Read the model definition and answer for the solid it produces. Units are mm, in the model's axes. Face numbers are marked on the shaded views. Give positions to 0.01 mm unless a question says otherwise; leave off trailing zeros. Order: outer loops, then holes, each group sorted by start corner. A loop starts at its lowest first (then second) coordinate and runs counter-clockwise, first axis right, second up. Notation, with made-up numbers: (3.25, -4) - (8.25, -4) arc R35 cw to (8.25, 34) - close; hole circle Ø4 at (48, 79). An arc over 180 degrees is marked (long way). One line per item, written item: value. Start each with the question number.
```python
from build123d import *

# Parameters (mm, degrees)
CROQUIS1_R              = 1.55
CROQUIS1_R_2            = 4
SALIENTE_EXTRUIR1_DEPTH = 120
CORTAR_EXTRUIR1_DEPTH   = 117
SALIENTE_EXTRUIR2_DEPTH = 10
CHAFL_N2_SIZE           = 3
CORTAR_EXTRUIR2_REACH   = 138.325
CROQUIS4_R              = 1.55
CHAFL_N3_SIZE           = 0.5
CORTAR_EXTRUIR3_START   = -2.5
CORTAR_EXTRUIR3_DEPTH   = 10
MATRIZC5_COUNT          = 8
CHAFL_N1_SIZE           = 2
CHAFL_N4_SIZE           = 0.5


with BuildPart() as part:
    # Croquis1 → Saliente-Extruir1 (new body)
    with BuildSketch(Plane(origin=(0, 0, 0), x_dir=(1, 0, 0), z_dir=(0, 1, 0))):
        Polygon((17, -7.04163056), (17, 7.04163056), (7.04163056, 17), (-7.04163056, 17), (-17, 7.04163056), (-17, -7.04163056), (-7.04163056, -17), (7.04163056, -17), align=None)
        with Locations(Location((0, 11, 0), (0, 0, 270))):
            Circle(CROQUIS1_R, mode=Mode.SUBTRACT)
        with Locations(Location((0, 0, 0), (0, 0, 270))):
            Circle(CROQUIS1_R_2, mode=Mode.SUBTRACT)
        with Locations(Location((7.778174593, 7.778174593, 0), (0, 0, 270))):
            Circle(CROQUIS1_R, mode=Mode.SUBTRACT)
        with Locations(Location((11, 0, 0), (0, 0, 270))):
            Circle(CROQUIS1_R, mode=Mode.SUBTRACT)
        with Locations(Location((7.778174593, -7.778174593, 0), (0, 0, 270))):
            Circle(CROQUIS1_R, mode=Mode.SUBTRACT)
        with Locations(Location((0, -11, 0), (0, 0, 270))):
            Circle(CROQUIS1_R, mode=Mode.SUBTRACT)
        with Locations(Location((-7.778174593, -7.778174593, 0), (0, 0, 270))):
            Circle(CROQUIS1_R, mode=Mode.SUBTRACT)
        with Locations(Location((-11, 0, 0), (0, 0, 270))):
            Circle(CROQUIS1_R, mode=Mode.SUBTRACT)
        with Locations(Location((-7.778174593, 7.778174593, 0), (0, 0, 270))):
            Circle(CROQUIS1_R, mode=Mode.SUBTRACT)
    extrude(amount=SALIENTE_EXTRUIR1_DEPTH)

    # Croquis2 → Cortar-Extruir1 (cut)
    with BuildSketch(Plane(origin=(0, 120, 0), x_dir=(1, 0, 0), z_dir=(0, 1, 0))):
        Polygon((6.213203436, 15), (-6.213203436, 15), (-15, 6.213203436), (-15, -6.213203436), (-6.213203436, -15), (6.213203436, -15), (15, -6.213203436), (15, 6.213203436), align=None)
    extrude(amount=-CORTAR_EXTRUIR1_DEPTH, mode=Mode.SUBTRACT)

    # Croquis3 → Saliente-Extruir2 (add)
    with BuildSketch(Plane(origin=(0, 120, 0), x_dir=(1, 0, 0), z_dir=(0, 1, 0))):
        Polygon((7.04163056, 17), (-7.04163056, 17), (-17, 7.04163056), (-17, -7.04163056), (-7.04163056, -17), (7.04163056, -17), (17, -7.04163056), (17, 7.04163056), align=None)
        Polygon((12, -4.970562748), (12, 4.970562748), (4.970562748, 12), (-4.970562748, 12), (-12, 4.970562748), (-12, -4.970562748), (-4.970562748, -12), (4.970562748, -12), align=None, mode=Mode.SUBTRACT)
    extrude(amount=SALIENTE_EXTRUIR2_DEPTH)

    # Chaflán2
    chafl_n2_edges = [part.edges().sort_by_distance(p)[0] for p in [
        (10.606601718, 120, -10.606601718),
        (0, 120, -15),
        (-10.606601718, 120, -10.606601718),
        (-15, 120, 0),
        (-10.606601718, 120, 10.606601718),
        (0, 120, 15),
        (10.606601718, 120, 10.606601718),
        (15, 120, 0),
    ]]
    chamfer(chafl_n2_edges, length=CHAFL_N2_SIZE - 0.0001)  # a hair under: the kernel refuses the full size

    # Croquis4 → Cortar-Extruir2 (cut, up to next)
    with BuildSketch(Plane(origin=(-12.02081528, 0, -12.02081528), x_dir=(-0.7071067811865472, 0, 0.7071067811865478), z_dir=(-0.7071067811865478, 0, -0.7071067811865472)), mode=Mode.PRIVATE) as cortar_extruir2_sk1:
        with Locations((0, 125)):
            Circle(CROQUIS4_R)
    cortar_extruir2_tool1 = extrude(cortar_extruir2_sk1.sketch, amount=-CORTAR_EXTRUIR2_REACH, mode=Mode.PRIVATE) & part.part
    cortar_extruir2 = cortar_extruir2_tool1.solids().sort_by_distance((-12.020815, 125, -12.020815))[0]
    add(cortar_extruir2, mode=Mode.SUBTRACT)

    # Chaflán3
    chafl_n3_edges = [part.edges().sort_by_distance(p)[0] for p in [
        (-10.924799769, 125, -13.116830791),
    ]]
    chamfer(chafl_n3_edges, length=CHAFL_N3_SIZE)

    # Croquis5 → Cortar-Extruir3 (cut)
    with BuildSketch(Plane(origin=(-12.02081528, 0, -12.02081528), x_dir=(-0.7071067811865471, 0, 0.7071067811865479), z_dir=(-0.7071067811865479, 0, -0.7071067811865471)).offset(CORTAR_EXTRUIR3_START)):
        Polygon((3.175426481, 125), (1.58771324, 127.75), (-1.58771324, 127.75), (-3.175426481, 125), (-1.58771324, 122.25), (1.58771324, 122.25), align=None)
    cortar_extruir3 = extrude(amount=-CORTAR_EXTRUIR3_DEPTH, mode=Mode.SUBTRACT)

    # MatrizC5: Cortar-Extruir2, Cortar-Extruir3 ×8 about axis
    matrizc5_axis = Axis((0, 0, 0), (0, 1, 0))
    add([cortar_extruir2.rotate(matrizc5_axis, i * 360 / MATRIZC5_COUNT) for i in range(1, MATRIZC5_COUNT)], mode=Mode.SUBTRACT)
    add([cortar_extruir3.rotate(matrizc5_axis, i * 360 / MATRIZC5_COUNT) for i in range(1, MATRIZC5_COUNT)], mode=Mode.SUBTRACT)

    # Chaflán1
    chafl_n1_edges = [part.edges().sort_by_distance(p)[0] for p in [
        (17, 0, 0),
        (12.02081528, 0, 12.02081528),
        (0, 0, 17),
        (-12.02081528, 0, 12.02081528),
        (-17, 0, 0),
        (-12.02081528, 0, -12.02081528),
        (0, 0, -17),
        (12.02081528, 0, -12.02081528),
    ]]
    chamfer(chafl_n1_edges, length=CHAFL_N1_SIZE)

    # Chaflán4
    chafl_n4_edges = [part.edges().sort_by_distance(p)[0] for p in [
        (12.02081528, 130, -12.02081528),
        (0, 130, -17),
        (-12.02081528, 130, -12.02081528),
        (-17, 130, 0),
        (-12.02081528, 130, 12.02081528),
        (0, 130, 17),
        (12.02081528, 130, 12.02081528),
        (17, 130, 0),
    ]]
    chamfer(chafl_n4_edges, length=CHAFL_N4_SIZE)


solid = part.part
```
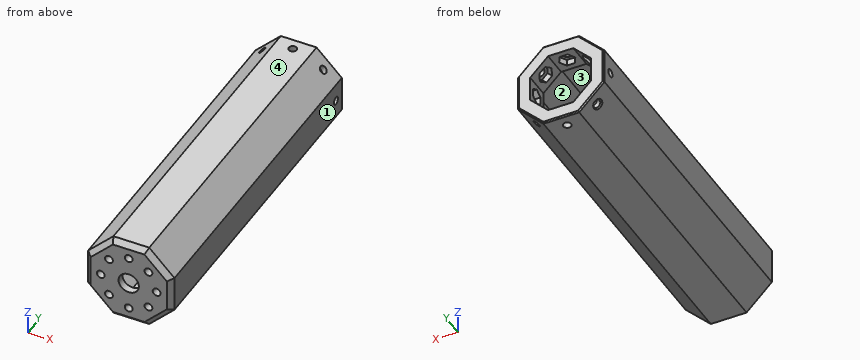
1) Each of these flat-tipped pins is pushed along its axis until it touches: pin 1 (1.9 mm diameter, centred on x = 0, z = -11, fed in from +Y); pin 2 (1.5 mm diameter, centred on x = -13, y = 59, fed in from +Z); pin 3 (1 mm diameter, centred on y = 61, z = -13, fed in from +X); pin 4 (1 mm diameter, centred on y = 102.5, z = -10.5, fed in from -X). Where does it stop, or does it pass through?
2) Section B-B on x = 0 is taken. Give the number of separate pieces and of enclosed holes in the cut face, plus the area to 3 significant figures.
3) The mould has two halves that part along X. Classify the marked faces 1, 2, 3 and 4: +X half, -X half, draft (parallel to the pull), parting line (faces both ways), or undercut.
4) Find the intervals of material crossed by probe 1 along X at (y, z) = (93, 3); probe 2 along Y at (x, z) = (-9.5, -0.5), in increasing order. Write a range as from..to.
5) Section A-A on y = 93 is taken. Write down the section's boundary in (x, z), plus the area to 3 significant figures.
Solved:
1. pin 1: passes through
1. pin 2: stops at z = 11.79
1. pin 3: stops at x = 11.54
1. pin 4: stops at x = -14.04
2. separate pieces: 6
2. enclosed holes: 0
2. area: 589 mm2
3. face 1: +X half
3. face 2: undercut
3. face 3: undercut
3. face 4: draft
4. probe 1: x = -17..-15, 15..17
4. probe 2: y = 0..3
5. outline: (-17, -7.04) - (-7.04, -17) - (7.04, -17) - (17, -7.04) - (17, 7.04) - (7.04, 17) - (-7.04, 17) - (-17, 7.04) - close; hole (-15, -6.21) - (-6.21, -15) - (6.21, -15) - (15, -6.21) - (15, 6.21) - (6.21, 15) - (-6.21, 15) - (-15, 6.21) - close
5. area: 212 mm2
